Drawing for the job (mm, zero at the part's lowest x, y, z). A direction names the side the tool comes from. Round coordinates to 2 decimals unless told otherwise and drop trailing zeros. Order: outer loops, then holes, each group sorted by start corner. A loop starts at its lowest first (then second) coordinate and runs counter-clockwise, first axis right, second up. Notation, with made-up numbers: M 71.25,43.25 L 84.25,43.25 A22 cw 84.25,57.25 Z; hole C -38,-32.5 d8. An arc over 180 degrees is marked long. One line per item, written item: value. Start each with the question number.
Item 1: Band-saw the part on D-D, the plane y = 2.25. Write the cut outline in (x, z), then the cut area to 3 significant figures.
Item 2: Tool access for the marked faces 1, 2, 3 and 4: list every direction of +Z, -Z, +X, -X, +Y, -Y with a clear straight run to the whole face (end or side of a thin tool).
Item 3: Band-saw the part on C-C, the plane z = 14.5. Write the cut outline in (x, y).
Item 4: Band-saw the part on A-A, the plane y = 3.7. Write the cut outline in (x, z), then the cut area to 3 significant figures.
Item 5: Band-saw the part on B-B, the plane x = 3.7. Write the cut outline in (y, z).
Item 6: Pin check, flat tips, straight feed: pin 1 (3 mm diameter, centred on x = 5.5, z = 14, fed in from -Y); pin 2 (1.8 mm diameter, centred on x = 3.5, z = 4, fed in from -Y); pin 3 (1.5 mm diameter, centred on y = 2.5, z = 11, fed in from +X). Stop position of each tip, or through.
Item 7: Probe L1, parallel to Z at x = 7.25, y = 3.5; L2, parallel to Z at x = 4.25, y = 2; L3, parallel to X at y = 3.75, z = 24. List the from-to ranges inside material, lowest first.
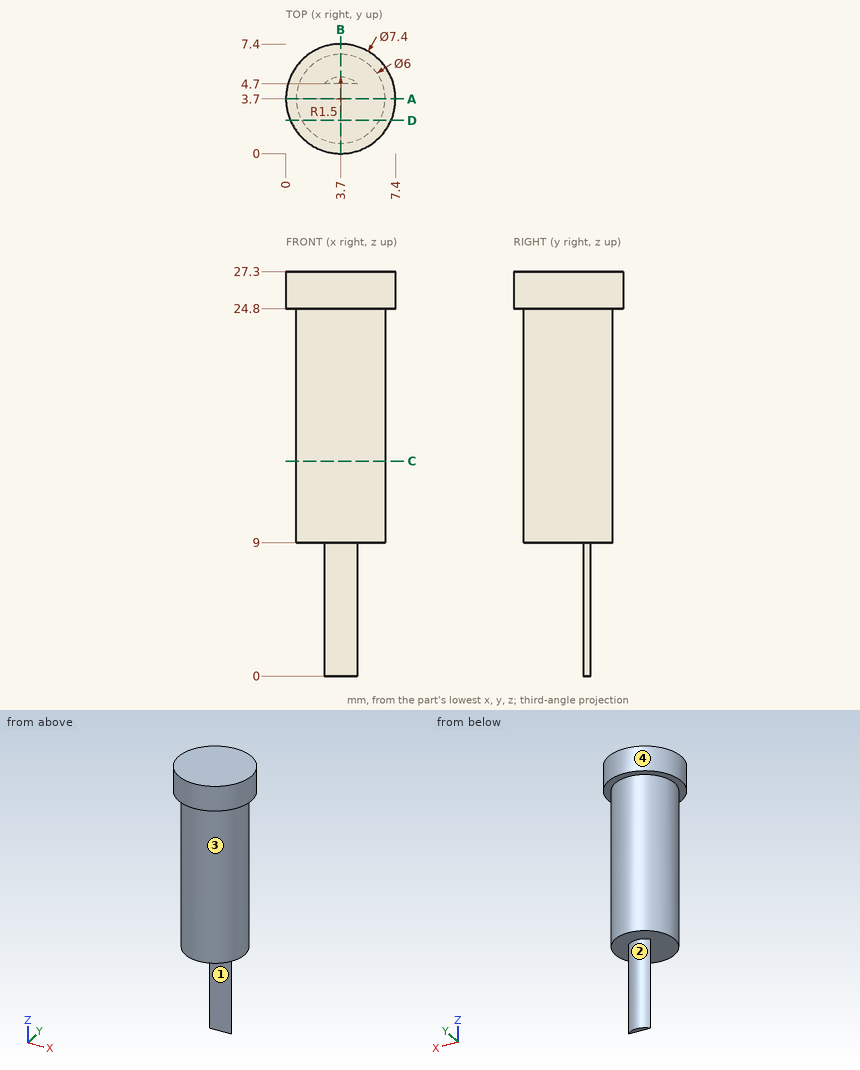
Output:
1. outline: M 0.3,24.8 L 1.07,24.8 L 1.07,9 L 6.33,9 L 6.33,24.8 L 7.1,24.8 L 7.1,27.3 L 0.3,27.3 Z
1. area: 100 mm²
2. face 1: -Z, +X, -X, -Y
2. face 2: -Z, +Y
2. face 3: -Z
2. face 4: +Z, -Z
3. outline: C 3.7,3.7 d6
4. outline: M 0,24.8 L 0.7,24.8 L 0.7,9 L 6.7,9 L 6.7,24.8 L 7.4,24.8 L 7.4,27.3 L 0,27.3 Z
4. area: 113 mm²
5. outline: M 0,24.8 L 0.7,24.8 L 0.7,9 L 4.7,9 L 4.7,0 L 5.2,0 L 5.2,9 L 6.7,9 L 6.7,24.8 L 7.4,24.8 L 7.4,27.3 L 0,27.3 Z
6. pin 1: stops at y = 0.72
6. pin 2: stops at y = 4.7
6. pin 3: stops at x = 6.67
7. L1: z = 24.8 to 27.3
7. L2: z = 9 to 27.3
7. L3: x = 0.7 to 6.7
